from build123d import *

# Parameters (mm, degrees)
F1_DEPTH = 52
F3_R     = 25.99999
F2_R     = 11
F4_DEPTH = 38
F5_DEPTH = 38


# Not quite as in the source:
# - a fillet or chamfer is up to 0.001 mm smaller than in the source, because OpenCascade refuses the exact size


with BuildPart() as f1:
    # F0 (on Front) → F1 (new body)
    with BuildSketch(Plane.XZ):
        with BuildLine():
            Line((46.2857175011, 0), (156.2857175011, 0))
            Line((156.2857175011, 0), (156.2857175011, 38))
            Line((156.2857175011, 38), (35.4412569068, 38))
            ThreePointArc((35.4412569068, 38), (-45.4728396677, 69.2358246763), (-97.7142824989, 0))
            Line((-97.7142824989, 0), (-67.7142824989, 0))
            ThreePointArc((-67.7142824989, 0), (-25.7142824989, 42), (16.2857175011, 0))
            Line((16.2857175011, 0), (46.2857175011, 0))
        make_face()
    extrude(amount=F1_DEPTH)

    # F3 (radius 26 in the source; OpenCascade refuses exactly that, so slightly less here)
    f3_edges = [f1.edges().sort_by_distance(p)[0] for p in [
        (156.285718, 0, 19),
        (156.285718, -52, 19),
    ]]
    fillet(f3_edges, radius=F3_R)

    # F2 (on face) → F4 (cut)
    with BuildSketch(Plane.XY.offset(38)):
        with Locations((130.2857175011, -26)):
            Circle(F2_R)
    extrude(amount=-F4_DEPTH, mode=Mode.SUBTRACT)

    # F2 (on face) → F5 (cut)
    with BuildSketch(Plane.XY.offset(38)):
        with Locations((82.2857175011, -26)):
            Circle(F2_R)
    extrude(amount=-F5_DEPTH, mode=Mode.SUBTRACT)

    # F6 (on face) → F7 (revolve, cut)
    with BuildSketch(Plane(origin=(0, 0, 0), x_dir=(1, 0, 0), z_dir=(0, 0, -1))):
        Polygon((-25.6639542129, 52), (-85.6639542129, 52), (-67.6639542129, 0), (-25.6639542129, 0), align=None)
    revolve(axis=Axis((-25.6639542129, -26, 0), (0, -1, 0)), mode=Mode.SUBTRACT)


solid = f1.part
Can you work these out from the model? Positions are in its coordinate system, mm. A direction names the side the tool comes from. Coordinates: 2 decimals unless noted, no trailing zeros. Loops run counter-clockwise (first coordinate to the right, second up) from the corner with the lowest first, then second, coordinate; pieces in that order, holes last. Notation, with made-up numbers: M 15,-24 L 46,-24 A34 cw 46,14 Z; hole C -13.75,86.25 d7. An arc over 180 degrees is marked long. Answer as CSV lines item,"result". Start each with the question number.
1. Suppose I cut it at A-A, the plane x = 127. List the corners of the cut face in (y, z) for me, plus the area to 3 significant figures.
2. Thinking about a two-plate mould opening in Y: for faces 1 (the face through (127.9, -36.74, 19.27)), 2 (the face through (-24.589, -19.858, 48.862)), 3 (the face through (-86, -20, 0)), 4 (the face through (79.9, -36.74, 19.27)), which applies, +Y half, -Y half, draft (parallel to the pull), parting line (faces both ways), or undercut?
3. Suppose I cut it at B-B, the plane z = 21. Count the separate pieces of the cut face and the enclosed holes in it, plus the area to 3 significant figures.
4. For faces 5 (the face through (85, -14, 0)), 6 (the face through (97, -26, 38)), which set-ups out of +Z, -Z, +X, -X, +Y, -Y let a thin tool reach every point of the face, with its end or its side?
5. If I drill on probe 1 along Z at (x, y) = (99, -13); probe 2 along X at (y, z) = (-33, 24.5); probe 3 along Z at (x, y) = (-25, -4), over which ranges is the centre line in solid material (lowest first)? Write a range as [from, to].
6. For pin 1 Ø2 at (y, z) = (-21, 37.5) entering from +X; pin 2 Ø4 at (y, z) = (-11.5, 52.5) entering from -X; pin 3 Ø12 at (x, y) = (109.5, -43) entering from +Z, each with a flat end and sliding along its axis, tell me the tip position at first contact or that it passes through.
7. Suppose I cut it at C-C, the plane y = -8.5. List the corners of the cut face in (x, z) for me, plus the area to 3 significant figures.
Output:
1,outline,"M -52,0 L -36.5,0 L -36.5,38 L -52,38 Z; M -15.5,0 L 0,0 L 0,38 L -15.5,38 Z"
1,area,"1,180 mm^2"
2,face 1,"undercut"
2,face 2,"-Y half"
2,face 3,"draft"
2,face 4,"undercut"
3,separate pieces,"2"
3,enclosed holes,"2"
3,area,"7,170 mm^2"
4,face 5,"-Z, +X, -X, +Y, -Y"
4,face 6,"+Z, +X, +Y, -Y"
5,probe 1,"z = [0, 38]"
5,probe 2,"x = [-93.42, -73.14], [21.81, 73.8], [90.77, 121.8], [138.77, 155.33]"
5,probe 3,"z = [43.38, 72]"
6,pin 1,"stops at x = 155.98"
6,pin 2,"stops at x = -77.03"
6,pin 3,"stops at z = 38"
7,outline,"M -97.71,0 L -70.61,0 A44.94 cw 19.28,0 L 149.51,0 L 149.51,38 L 35.44,38 A72 ccw Z"
7,area,"9,030 mm^2"
